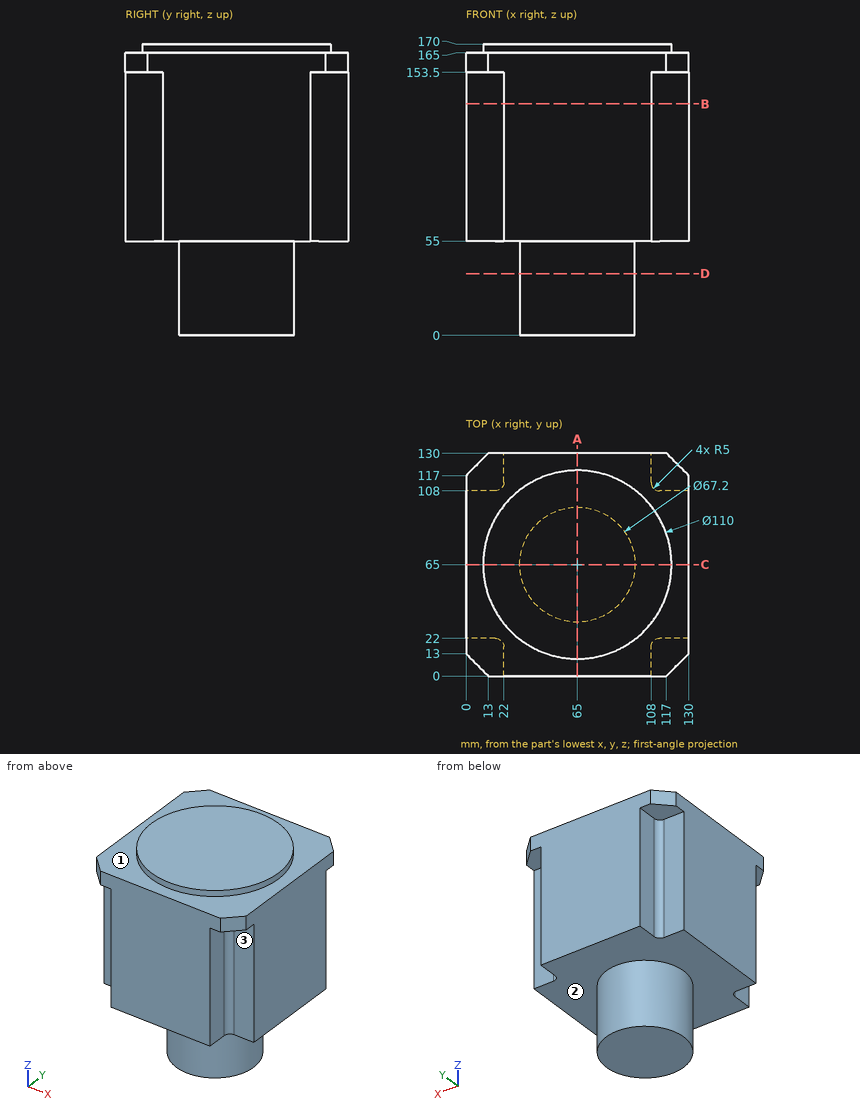
Verification items for this drawing (mm, ordinates from the low corner). A direction names the side the tool comes from. Give positions to 0.01 mm unless a question says otherwise; leave off trailing zeros. Loops run counter-clockwise (first coordinate to the right, second up) from the corner with the lowest first, then second, coordinate; pieces in that order, holes last. Notation, with made-up numbers: M 7.25,40.5 L 52.25,40.5 A15 cw 52.25,51.5 Z; hole C 72,19 d11. An arc over 180 degrees is marked long. Return JSON: item names as keys, results as strings. Group by question number.
1. Thickness scan on L1, parallel to Z at x = 109, y = 125.5; L2, parallel to Z at x = 49, y = 115.5; L3, parallel to X at y = 116, z = 99.5. Record the ranges inside material, lowest first.
2. Go/stop test with flat-tipped pins: pin 1 (8.5 mm diameter, centred on x = 124, z = 85.5, fed in from -Y); pin 2 (17.5 mm diameter, centred on x = 5.5, y = 116.5, fed in from -Z); pin 3 (3 mm diameter, centred on x = 59.5, z = 20.5, fed in from -Y); pin 4 (10 mm diameter, centred on x = 109, z = 59, fed in from -Y). Record where each tip stops, or that it passes through.
3. Cross-section at A-A on x = 65. Record the boundary of the cut face in (y, z).
4. Cross-section at D-D on z = 36. Record the boundary of the cut face in (x, y), plus the area to 3 significant figures.
5. Tool access check on the marked faces 1, 2 and 3. Record the directions out of +Z, -Z, +X, -X, +Y, -Y that give a thin tool (end or side, any length) a straight path to the whole face; none if there is none.
6. Cross-section at B-B on z = 135. Record the boundary of the cut face in (x, y), plus the area to 3 significant figures.
Return value:
{
 "1": {"L1": "153.5 to 165", "L2": "55 to 170", "L3": "22 to 108"},
 "2": {"pin 1": "y = 22", "pin 2": "z = 55", "pin 3": "y = 31.64", "pin 4": "y = 0"},
 "3": {"outline": "M 0,55 L 31.4,55 L 31.4,0 L 98.6,0 L 98.6,55 L 130,55 L 130,165 L 120,165 L 120,170 L 10,170 L 10,165 L 0,165 Z"},
 "4": {"outline": "C 65,65 d67.2", "area": "3,550 mm^2"},
 "5": {"face 1": "+Z", "face 2": "-Z", "face 3": "-Z, +X, -Y"},
 "6": {"outline": "M 0,22 L 17,22 A5 cw 22,17 L 22,0 L 108,0 L 108,17 A5 cw 113,22 L 130,22 L 130,108 L 113,108 A5 cw 108,113 L 108,130 L 22,130 L 22,113 A5 cw 17,108 L 0,108 Z", "area": "15,000 mm^2"}
}
